Read the model definition and answer for the solid it produces. Units are mm, in the model's axes. Coordinates: 2 decimals unless noted, no trailing zeros. Write each loop counter-clockwise with the first axis right and the second up, starting at its lowest first coordinate (ties: lowest second). Pieces come first, ordered by that corner, then holes. Notation, with made-up numbers: (23, -11.5) - (45, -11.5) arc R22 cw to (45, 18.5) - close; hole circle Ø6 at (-14.75, -11). An arc over 180 degrees is marked (long way). Use a Markdown table: item, result.
from build123d import *

# Parameters (mm, degrees)
BOSS_EXTRUDE1_DEPTH = 5
CUT_EXTRUDE1_START  = 5
SKETCH2_R           = 2.45
CUT_EXTRUDE1_DEPTH  = 4
SKETCH3_R           = 1.5
BOSS_EXTRUDE2_DEPTH = 3


with BuildPart() as part:
    # Sketch1 → Boss-Extrude1 (new body)
    with BuildSketch(Plane(origin=(0, 0, 0), x_dir=(1, 0, 0), z_dir=(0, 1, 0))):
        Polygon((1.443375673, -2.5), (2.886751346, 0), (1.443375673, 2.5), (-1.443375673, 2.5), (-2.886751346, 0), (-1.443375673, -2.5), align=None)
    extrude(amount=BOSS_EXTRUDE1_DEPTH)

    # Sketch2 → Cut-Extrude1 (cut)
    with BuildSketch(Plane(origin=(0, 0, 0), x_dir=(1, 0, 0), z_dir=(0, 1, 0)).offset(CUT_EXTRUDE1_START)):
        with Locations(Location((0, 0, 0), (0, 0, 270))):
            Circle(SKETCH2_R)
    extrude(amount=-CUT_EXTRUDE1_DEPTH, mode=Mode.SUBTRACT)

    # Sketch3 → Boss-Extrude2 (add)
    with BuildSketch(Plane(origin=(0, 0, 0), x_dir=(1, 0, 0), z_dir=(0, 1, 0))):
        with Locations(Location((0, 0, 0), (0, 0, 270))):
            Circle(SKETCH3_R)
    extrude(amount=-BOSS_EXTRUDE2_DEPTH)


solid = part.part
(1) A cutting plane is placed at C-C, the plane z = -1.9. Write down the section's boundary in (x, y), and give its area (3 significant figures).
Report:
| item | result |
|---|---|
| outline | (-1.79, 0) - (1.79, 0) - (1.79, 5) - (1.55, 5) - (1.55, 1) - (-1.55, 1) - (-1.55, 5) - (-1.79, 5) - close |
| area | 5.52 mm² |
(2) A cutting plane is placed at B-B, the plane x = 0. Write down the section's boundary in (y, z), and give its area (3 significant figures).
Report:
| item | result |
|---|---|
| outline | (-3, -1.5) - (0, -1.5) - (0, -2.5) - (5, -2.5) - (5, -2.45) - (1, -2.45) - (1, 2.45) - (5, 2.45) - (5, 2.5) - (0, 2.5) - (0, 1.5) - (-3, 1.5) - close |
| area | 14.4 mm² |
(3) A cutting plane is placed at D-D, the plane y = -1.25. Write down the section's boundary in (x, z), and give its area (3 significant figures).
Report:
| item | result |
|---|---|
| outline | circle Ø3 at (0, 0) |
| area | 7.07 mm² |
(4) The mould has two halves that part along X. Classify faces 1 (the flat face through (1.24, 0, -1.15)), 2 (the cylindrical face through (0.736, 3.028, 2.337)), 3 (the cylindrical face through (0.45, -1.48, 1.43)), 4 (the flat face through (0, 1, 0)): pulls with the +X half, pulls with the -X half, needs draft (parallel to the pull), parting line crosses it, or undercut.
Report:
| item | result |
|---|---|
| face 1 | needs draft |
| face 2 | undercut |
| face 3 | parting line crosses it |
| face 4 | undercut |
(5) Each of these flat-tipped pins is pushed along its axis until it touches: P1, Ø3, axis at x = 2, y = -2, coming from the +Z side; P2, Ø3, axis at y = -1, z = 2, coming from the +X side; P3, Ø3, axis at x = 0, z = 0, coming from the +Y side. Where does it stop, or does it pass through?
Report:
| item | result |
|---|---|
| P1 | stops at z = 1.41 |
| P2 | stops at x = 2.38 |
| P3 | stops at y = 1 |
(6) A cutting plane is placed at A-A, the plane y = 4.25. Write down the section's boundary in (x, z).
Report:
| item | result |
|---|---|
| outline | (-2.89, 0) - (-1.44, -2.5) - (1.44, -2.5) - (2.89, 0) - (1.44, 2.5) - (-1.44, 2.5) - close; hole circle Ø4.9 at (0, 0) |
(7) Straight lines are drawn through the part: L1, parallel to Y at x = -0.6, z = 1; L2, parallel to Y at x = 1.55, z = 1.3; L3, parallel to X at y = 4, z = 2.15. For each, find the intervals that lie inside material, in ascending order.
Report:
| item | result |
|---|---|
| L1 | y = -3 to 1 |
| L2 | y = 0 to 1 |
| L3 | x = -1.65 to -1.17, 1.17 to 1.65 |
